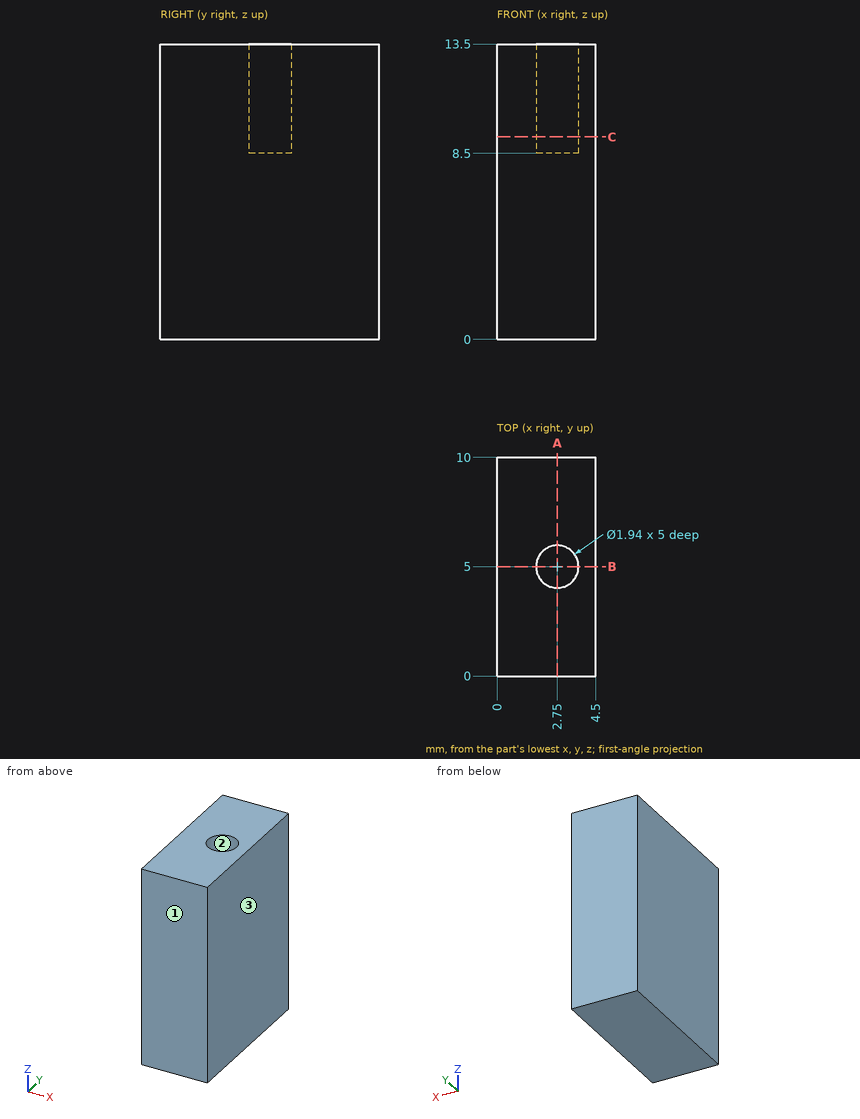
The drawing under review shows one solid part. Ordinate dimensions are in mm from its lowest x, y, z. Give positions to 0.01 mm unless a question says otherwise; leave off trailing zeros. Loops run counter-clockwise (first coordinate to the right, second up) from the corner with the lowest first, then second, coordinate; pieces in that order, holes last. Notation, with made-up numbers: M -35,-39.75 L 10,-39.75 A14 cw 10,-27.75 Z; hole C 78,49.25 d7. An arc over 180 degrees is marked long. Return JSON: item names as keys, results as strings. Group by question number.
Item 1: For probe 1 along Y at (x, z) = (2.75, 11.5); probe 2 along Y at (x, z) = (2.4, 13.25); probe 3 along Z at (x, y) = (2.65, 4.25), list the stretches that pass through material, from the lowest coordinate up.
Item 2: We need section A-A (x = 2.75). Give the boundary of the cut face in (y, z).
Item 3: We need section C-C (z = 9.25). Give the boundary of the cut face in (x, y).
Item 4: We need section B-B (y = 5). Give the boundary of the cut face in (x, z).
Item 5: Mouldability with a two-part tool opening along Y and no side actions: class the marked faces 1, 2 and 3 as released by +Y, released by -Y, zero draft, split by the parting line, or undercut.
Output:
{
 "1": {"probe 1": "y = 0 to 4.03, 5.97 to 10", "probe 2": "y = 0 to 4.1, 5.9 to 10", "probe 3": "z = 0 to 8.5"},
 "2": {"outline": "M 0,0 L 10,0 L 10,13.5 L 5.97,13.5 L 5.97,8.5 L 4.03,8.5 L 4.03,13.5 L 0,13.5 Z"},
 "3": {"outline": "M 0,0 L 4.5,0 L 4.5,10 L 0,10 Z; hole C 2.75,5 d1.94"},
 "4": {"outline": "M 0,0 L 4.5,0 L 4.5,13.5 L 3.72,13.5 L 3.72,8.5 L 1.78,8.5 L 1.78,13.5 L 0,13.5 Z"},
 "5": {"face 1": "released by -Y", "face 2": "undercut", "face 3": "zero draft"}
}
